Source: CAD feature listing. Evaluate the final solid. Frame: model axes, mm. A direction names the side the tool comes from. Give positions to 0.01 mm unless a question says otherwise; leave off trailing zeros. Order: outer loops, then holes, each group sorted by start corner. A loop starts at its lowest first (then second) coordinate and runs counter-clockwise, first axis right, second up. Notation, with made-up numbers: M 87.5,88.25 L 106.5,88.25 A18 ccw 106.5,93.25 Z; hole C 25.5,11.5 d10. An arc over 180 degrees is marked long. Return JSON: item names as keys, results as strings.
from build123d import *

# Parameters (mm, degrees)
F0_R     = 12.7
F1_DEPTH = 76.2
F4_D     = 3.302
F4_DEPTH = 12.7
F4_TIP   = 0.992020882


with BuildPart() as f1:
    # F0 (on Right) → F1 (new body)
    with BuildSketch(Plane.YZ):
        with BuildLine():
            Line((19.05, -25.4), (19.05, 0))
            ThreePointArc((19.05, 0), (0, 19.05), (-19.05, 0))
            Line((-19.05, 0), (-19.05, -25.4))
            Line((-19.05, -25.4), (19.05, -25.4))
        make_face()
        Circle(F0_R, mode=Mode.SUBTRACT)
    extrude(amount=F1_DEPTH)

    # F4
    with Locations(Plane(origin=(0, 0, -25.4), x_dir=(1, 0, 0), z_dir=(0, 0, -1))):
        with Locations((6.35, 12.7), (6.35, -12.7), (69.85, -12.7), (69.85, 12.7)):
            Hole(F4_D / 2, depth=F4_DEPTH)
            with Locations((0, 0, -(F4_DEPTH + F4_TIP / 2))):  # 118° drill point
                Cone(0, F4_D / 2, F4_TIP, mode=Mode.SUBTRACT)


solid = f1.part
1. Section query C-C (x = 62.5). Return loops of the section in (y, z), then the cut area to 3 significant figures.
Evaluation:
{"outline": "M -19.05,-25.4 L 19.05,-25.4 L 19.05,0 A19.05 ccw -19.05,0 Z; hole C 0,0 d25.4", "area": "1,030 mm^2"}
2. Section query B-B (z = -7). Return loops of the section in (x, y), then the cut area to 3 significant figures.
Evaluation:
{"outline": "M 0,-19.05 L 76.2,-19.05 L 76.2,-10.6 L 0,-10.6 Z; M 0,10.6 L 76.2,10.6 L 76.2,19.05 L 0,19.05 Z", "area": "1,290 mm^2"}
3. First-contact query: pin 1 (4.5 mm diameter, centred on x = 69.85, y = -12.7, fed in from +Z); pin 2 (1.5 mm diameter, centred on x = 46, z = 2, fed in from -Y); pin 3 (5.5 mm diameter, centred on x = 6.35, y = -12.7, fed in from +Z) (3 decimals). Flat tips, straight axial feed; report the tip coordinate or a pass-through.
Evaluation:
{"pin 1": "stops at z = 15.93", "pin 2": "stops at y = -19.01", "pin 3": "stops at z = 16.245"}
4. Section query D-D (z = 16). Return loops of the section in (x, y), then the cut area to 3 significant figures.
Evaluation:
{"outline": "M 0,-10.34 L 76.2,-10.34 L 76.2,10.34 L 0,10.34 Z", "area": "1,580 mm^2"}
5. Draft query along Y for faces 1 (the face through (0, 0, -13)), 2 (the face through (7.66, 13.705, -18.961)), 3 (the face through (37.567, 0.419, 19.045)). Return one class per face: pulls with the +Y half, pulls with the -Y half, needs draft (parallel to the pull), parting line crosses it, or undercut.
Evaluation:
{"face 1": "needs draft", "face 2": "undercut", "face 3": "parting line crosses it"}
6. Ray query, probe 1 along X at (y, z) = (-12.7, -22.5); probe 2 along Y at (x, z) = (6.35, -15.5); probe 3 along Y at (x, z) = (69, -22). Return the intervals inside material, ascending.
Evaluation:
{"probe 1": "x = 0 to 4.7, 8 to 68.2, 71.5 to 76.2", "probe 2": "y = -19.05 to -14.35, -11.05 to 11.05, 14.35 to 19.05", "probe 3": "y = -19.05 to -14.12, -11.28 to 11.28, 14.12 to 19.05"}
7. Set-up query: faces 4 (the face through (38, 19.05, -13)), 5 (the face through (6.565, -14.337, -18.961)). Return all of +Z, -Z, +X, -X, +Y, -Y with unobstructed straight access to the full face (end or side cutting, diameter ignored); none if empty.
Evaluation:
{"face 4": "+Z, -Z, +X, -X, +Y", "face 5": "-Z"}
8. Section query A-A (y = 0). Return loops of the section in (x, z).
Evaluation:
{"outline": "M 0,-25.4 L 76.2,-25.4 L 76.2,-12.7 L 0,-12.7 Z; M 0,12.7 L 76.2,12.7 L 76.2,19.05 L 0,19.05 Z"}
